```python
from build123d import *

# Parameters (mm, degrees)
CUT_EXTRUDE1_DEPTH      = 121.271567712
CUT_EXTRUDE1_DEPTH_BACK = 121.271567712
SKETCH1_6_W             = 6
SKETCH1_6_H             = 20
CUT_EXTRUDE2_DEPTH      = 24
SKETCH3_R               = 4
CUT_EXTRUDE3_DEPTH      = 114.258419555
CUT_EXTRUDE4_DEPTH      = 25
CUT_EXTRUDE4_DEPTH_BACK = 7


with BuildPart() as part:
    # Sketch1 one side → Revolve2 (revolve)
    with BuildSketch(Plane.XY):
        Polygon((0, 28.5), (0, 0), (20, 0), (20, 6.295), (45, 6.295), (45, 14.225), (99.878679656, 14.225), (102, 16.346320344), (102, 28.5), align=None)
    revolve(axis=Axis((0, 28.5, 0), (1, 0, 0)))

    # Sketch1_6 → Cut-Extrude1 (cut, two sides: drawn at the far end of the back side and taken through both)
    with BuildSketch(Plane.XY.offset(-CUT_EXTRUDE1_DEPTH_BACK)):
        with Locations((3, 28.5)):
            Rectangle(SKETCH1_6_W, SKETCH1_6_H)
    extrude(amount=CUT_EXTRUDE1_DEPTH + CUT_EXTRUDE1_DEPTH_BACK, mode=Mode.SUBTRACT)

    # Sketch2 → Cut-Extrude2 (cut)
    with BuildSketch(Plane(origin=(102, 0, 0), x_dir=(0, 0, -1), z_dir=(1, 0, 0))):
        with BuildLine():
            ThreePointArc((3.496044793, 40.14), (0, 40.653679656), (-3.496044793, 40.14))
            Line((-3.496044793, 40.14), (3.496044793, 40.14))
        make_face()
        with BuildLine():
            ThreePointArc((8.263535865, 40.14), (0, 42.775), (-8.263535865, 40.14))
            Line((-8.263535865, 40.14), (-3.496044793, 40.14))
            ThreePointArc((-3.496044793, 40.14), (0, 40.653679656), (3.496044793, 40.14))
            Line((3.496044793, 40.14), (8.263535865, 40.14))
        make_face()
        with BuildLine():
            Line((-3.496044793, 16.86), (-8.263535865, 16.86))
            ThreePointArc((-8.263535865, 16.86), (0, 14.225), (8.263535865, 16.86))
            Line((8.263535865, 16.86), (3.496044793, 16.86))
            ThreePointArc((3.496044793, 16.86), (0, 16.346320344), (-3.496044793, 16.86))
        make_face()
        with BuildLine():
            Line((3.496044793, 16.86), (-3.496044793, 16.86))
            ThreePointArc((-3.496044793, 16.86), (0, 16.346320344), (3.496044793, 16.86))
        make_face()
    extrude(amount=-CUT_EXTRUDE2_DEPTH, mode=Mode.SUBTRACT)

    # Sketch3 → Cut-Extrude3 (cut, through all)
    with BuildSketch(Plane(origin=(0, 40.14, 0), x_dir=(1, 0, 0), z_dir=(0, 1, 0))):
        with Locations(Location((90, 0, 0), (0, 0, 180))):
            Circle(SKETCH3_R)
    extrude(amount=-CUT_EXTRUDE3_DEPTH, mode=Mode.SUBTRACT)

    # Sketch4 → Cut-Extrude4 (cut, two sides: drawn at the far end of the back side and taken through both)
    with BuildSketch(Plane(origin=(20, 0, 0), x_dir=(0, 0, -1), z_dir=(1, 0, 0)).offset(-CUT_EXTRUDE4_DEPTH_BACK)):
        with BuildLine():
            ThreePointArc((19.267848868, 49.5), (0, 57), (-19.267848868, 49.5))
            Line((-19.267848868, 49.5), (-7.215401929, 49.5))
            ThreePointArc((-7.215401929, 49.5), (0, 50.705), (7.215401929, 49.5))
            Line((7.215401929, 49.5), (19.267848868, 49.5))
        make_face()
        with BuildLine():
            ThreePointArc((7.215401929, 49.5), (0, 50.705), (-7.215401929, 49.5))
            Line((-7.215401929, 49.5), (7.215401929, 49.5))
        make_face()
        with BuildLine():
            Line((7.215401929, 7.5), (-7.215401929, 7.5))
            ThreePointArc((-7.215401929, 7.5), (0, 6.295), (7.215401929, 7.5))
        make_face()
        with BuildLine():
            Line((-7.215401929, 7.5), (-19.267848868, 7.5))
            ThreePointArc((-19.267848868, 7.5), (0, 0), (19.267848868, 7.5))
            Line((19.267848868, 7.5), (7.215401929, 7.5))
            ThreePointArc((7.215401929, 7.5), (0, 6.295), (-7.215401929, 7.5))
        make_face()
    extrude(amount=CUT_EXTRUDE4_DEPTH + CUT_EXTRUDE4_DEPTH_BACK, mode=Mode.SUBTRACT)


solid = part.part
```
Build history of the part. All positions in model axes, mm. A direction names the side the tool comes from. Round coordinates to 2 decimals unless told otherwise and drop trailing zeros. Loops run counter-clockwise (first coordinate to the right, second up) from the corner with the lowest first, then second, coordinate; pieces in that order, holes last. Notation, with made-up numbers: M 21.5,80.25 L 27.5,80.25 A4 ccw 27.5,87.25 Z; hole C 61.5,-13 d2. An arc over 180 degrees is marked long. Answer as CSV lines item,"result".
1. Cut at C-C on y = 28.5. Write the cut outline in (x, z) (3 decimals).
Resolved:
outline,"M 6,-28.5 L 20,-28.5 L 20,-22.205 L 45,-22.205 L 45,-14.275 L 99.879,-14.275 L 102,-12.154 L 102,12.154 L 99.879,14.275 L 45,14.275 L 45,22.205 L 20,22.205 L 20,28.5 L 6,28.5 Z; hole C 90,0 d8"
2. Cut at D-D on y = 10. Write the cut outline in (x, z).
Resolved:
outline,"M 0,-21.68 L 20,-21.68 L 20,-12.28 L 45,-12.28 L 45,12.28 L 20,12.28 L 20,21.68 L 0,21.68 Z"
3. Flat gauge pins, fed straight in: P1, Ø9.5, axis at x = 24.5, z = 9.5, coming from the -Y side; P2, Ø5, axis at x = 77, z = 4.5, coming from the -Y side; P3, Ø8.5, axis at y = 51.5, z = -3, coming from the +X side. Where does each tip first touch, or does it go through?
Resolved:
P1,"stops at y = 7.5"
P2,"stops at y = 14.37"
P3,"stops at x = 45"
4. 3-axis set-ups, long thin cutter, end or side, ignore diameter. For faces 1 (the flat face through (78, 41, 0)), 2 (the flat face through (25, 7.5, 0)), 3 (the flat face through (3, 38.5, 0)): which of +Z, -Z, +X, -X, +Y, -Y reach the whole face in a straight line?
Resolved:
face 1,"+Z, -Z, +X, +Y"
face 2,"+Z, -Z, +X, -Y"
face 3,"+Z, -Z, -X"
5. Cut at A-A on z = 0. Write the cut outline in (x, y) (3 decimals), then the cut area to 3 significant figures.
Resolved:
outline,"M 0,0 L 13,0 L 13,7.5 L 45,7.5 L 45,14.225 L 78,14.225 L 78,16.86 L 86,16.86 L 86,40.14 L 78,40.14 L 78,42.775 L 45,42.775 L 45,49.5 L 13,49.5 L 13,57 L 0,57 L 0,38.5 L 6,38.5 L 6,18.5 L 0,18.5 Z; M 94,16.86 L 102,16.86 L 102,40.14 L 94,40.14 Z"
area,"3,280 mm²"
6. Two-plate mould, pull along Y, no slides. Class faces 4 (the cylindrical face through (94, 29, 0)), 5 (the flat face through (6, 28, 0)), 6 (the cylindrical face through (10.14, 2.173, 10.916)): released by +Y, released by -Y, zero draft, split by the parting line, or undercut.
Resolved:
face 4,"zero draft"
face 5,"undercut"
face 6,"split by the parting line"
7. Wall check: probe 1 along Z at (x, y) = (90, 29); probe 2 along X at (y, z) = (22, 14.5); probe 3 along Y at (x, z) = (94, -3). Give the ranges that are in metal, low to high. Write a range as [from, to].
Resolved:
probe 1,"z = [-14.27, -4], [4, 14.27]"
probe 2,"x = [6, 45]"
probe 3,"y = [16.86, 40.14]"
8. Cut at B-B on x = 90. Write the cut outline in (y, z) (3 decimals).
Resolved:
outline,"M 16.86,-8.264 A14.275 ccw 40.14,-8.264 L 40.14,-4 L 16.86,-4 Z; M 16.86,4 L 40.14,4 L 40.14,8.264 A14.275 ccw 16.86,8.264 Z"
